from build123d import *

# Parameters (mm, degrees)
F0_R     = 0.75
F1_DEPTH = 5
F2_R     = 1.575
F3_DEPTH = 5.001
F4_R     = 4.5
F5_DEPTH = 3
F6_R     = 2
F7_DEPTH = 2


with BuildPart() as f1:
    # F0 (on Top) → F1 (new body)
    with BuildSketch(Plane.XY):
        with BuildLine():
            Line((-8, 35), (-8, 0))
            Line((-8, 0), (-8, -35))
            ThreePointArc((-8, -35), (0, -43), (8, -35))
            Line((8, -35), (8, 0))
            Line((8, 0), (8, 35))
            ThreePointArc((8, 35), (0, 43), (-8, 35))
        make_face()
        with Locations((-2.969848, -37.969848)):
            Circle(F0_R, mode=Mode.SUBTRACT)
        with Locations((-2.969848, -32.030152)):
            Circle(F0_R, mode=Mode.SUBTRACT)
        with Locations((2.969848, -37.969848)):
            Circle(F0_R, mode=Mode.SUBTRACT)
        with Locations((2.969848, -32.030152)):
            Circle(F0_R, mode=Mode.SUBTRACT)
        with Locations((-2.969848, 32.030152)):
            Circle(F0_R, mode=Mode.SUBTRACT)
        with Locations((-2.969848, 37.969848)):
            Circle(F0_R, mode=Mode.SUBTRACT)
        with Locations((2.969848, 32.030152)):
            Circle(F0_R, mode=Mode.SUBTRACT)
        with Locations((2.969848, 37.969848)):
            Circle(F0_R, mode=Mode.SUBTRACT)
    extrude(amount=F1_DEPTH)

    # F2 (on face) → F3 (cut, through all)
    with BuildSketch(Plane.XY.offset(5)):
        with Locations((0, 5)):
            Circle(F2_R)
        with Locations((0, -5)):
            Circle(F2_R)
    extrude(amount=-F3_DEPTH, mode=Mode.SUBTRACT)

    # F4 (on face) → F5 (cut)
    with BuildSketch(Plane.XY.offset(5)):
        with Locations((0, 5)):
            Circle(F4_R)
        with Locations((0, -5)):
            Circle(F4_R)
    extrude(amount=-F5_DEPTH, mode=Mode.SUBTRACT)

    # F6 (on face) → F7 (cut)
    with BuildSketch(Plane(origin=(0, 0, 0), x_dir=(1, 0, 0), z_dir=(0, 0, -1))):
        with Locations((-2.969848, 37.969848)):
            Circle(F6_R)
        with Locations((2.969848, 37.969848)):
            Circle(F6_R)
        with Locations((2.969848, 32.030152)):
            Circle(F6_R)
        with Locations((-2.969848, 32.030152)):
            Circle(F6_R)
        with Locations((-2.969848, -32.030152)):
            Circle(F6_R)
        with Locations((-2.969848, -37.969848)):
            Circle(F6_R)
        with Locations((2.969848, -37.969848)):
            Circle(F6_R)
        with Locations((2.969848, -32.030152)):
            Circle(F6_R)
    extrude(amount=-F7_DEPTH, mode=Mode.SUBTRACT)


solid = f1.part
Input: part model. Units: mm. Frame: model coordinates. A direction names the side the tool comes from. Give positions to 0.01 mm unless a question says otherwise; leave off trailing zeros.
Q1. Ray query, probe 1 along Y at (x, z) = (-2.5, 1.55); probe 2 along Y at (x, z) = (3.75, 1.6); probe 3 along X at (y, z) = (38, 0.7). Return the intervals inside material, ascending.
Checked values:
probe 1: y = -42.6 to -39.91, -36.03 to -33.97, -30.09 to 30.09, 33.97 to 36.03, 39.91 to 42.6
probe 2: y = -42.07 to -39.81, -36.13 to -33.87, -30.19 to 30.19, 33.87 to 36.13, 39.81 to 42.07
probe 3: x = -7.42 to -4.97, -0.97 to 0.97, 4.97 to 7.42
Q2. Set-up query: faces 1 (the cylindrical face through (2.709, -39.953, 0.986)), 2 (the cylindrical face through (3.373, -37.337, 3.479)), 3 (the cylindrical face through (-0.98, -9.39, 3.52)). Return all of +Z, -Z, +X, -X, +Y, -Y with unobstructed straight access to the full face (end or side cutting, diameter ignored); none if empty.
Checked values:
face 1: -Z
face 2: +Z, -Z
face 3: +Z
Q3. Draft query along Y for faces 4 (the cylindrical face through (0, 43, 2)), 5 (the cylindrical face through (2.872, 32.774, 3.479)), 6 (the cylindrical face through (-0.21, 6.56, 1.01)), 7 (the flat face through (0, 1, 0)). Return one class per face: +Y half, -Y half, draft (parallel to the pull), parting line (faces both ways), or undercut.
Checked values:
face 4: +Y half
face 5: undercut
face 6: undercut
face 7: draft
Q4. Contact query for flat-ended pins moving along their axis: pin 1 Ø1.5 at (x, z) = (-3.5, 1) entering from +Y; pin 2 Ø1.9 at (x, y) = (0, -5) entering from +Z; pin 3 Ø1.2 at (x, y) = (2, 32.5) entering from -Z; pin 4 Ø3 at (x, z) = (-4, 4.5) entering from -Y. Output: stop coordinate, or through.
Checked values:
pin 1: stops at y = 42.51
pin 2: passes through
pin 3: stops at z = 2
pin 4: stops at y = -42.6
Q5. Section A-A on z = 3.05. State how many separate pieces and enclosed holes the cut face has, and give its area (3 significant figures).
Checked values:
separate pieces: 1
enclosed holes: 10
area: 1,180 mm2
